Verification items for the finished model (mm, model axes). A direction names the side the tool comes from. Coordinates: 2 decimals unless noted, no trailing zeros. Write each loop counter-clockwise with the first axis right and the second up, starting at its lowest first coordinate (ties: lowest second). Pieces come first, ordered by that corner, then holes. Notation, with made-up numbers: (61.25, -18.75) -> (79.25, -18.75) arc R12 cw to (79.25, -11.75) -> close; hole circle Ø11 at (-37, -13.5). An arc over 180 degrees is marked (long way). Answer in a Markdown table with one row per item.
```python
from build123d import *

# Parameters (mm, degrees)
F1_DEPTH = 50.8
F2_R     = 12.7
F4_D     = 12.7


with BuildPart() as f1:
    # F0 (on Top) → F1 (new body)
    with BuildSketch(Plane.XY):
        Polygon((0, 50.8), (0, 0), (152.4, 0), (152.4, 76.2), (101.6, 76.2), (101.6, 50.8), align=None)
    extrude(amount=F1_DEPTH)

    # F2
    f2_edges = [f1.edges().sort_by_distance(p)[0] for p in [
        (0, 25.4, 0),
        (76.2, 0, 0),
        (152.4, 38.1, 0),
        (127, 76.2, 0),
        (101.6, 63.5, 0),
        (50.8, 50.8, 0),
        (152.4, 0, 25.4),
        (0, 0, 25.4),
        (0, 50.8, 25.4),
        (152.4, 76.2, 25.4),
    ]]
    fillet(f2_edges, radius=F2_R)

    # F4 (through all)
    with Locations(Plane.XY.offset(50.8)):
        with Locations((50.8, 25.4), (101.6, 25.4)):
            Hole(F4_D / 2)


solid = f1.part
```
1. Sectioned sample at A-A, the plane y = 25.4. Record the cut outline in (x, z), and give its area (3 significant figures).
Findings below:
| item | result |
|---|---|
| outline | (0, 12.7) arc R12.7 ccw to (12.7, 0) -> (44.45, 0) -> (44.45, 50.8) -> (0, 50.8) -> close; (57.15, 0) -> (95.25, 0) -> (95.25, 50.8) -> (57.15, 50.8) -> close; (107.95, 0) -> (139.7, 0) arc R12.7 ccw to (152.4, 12.7) -> (152.4, 50.8) -> (107.95, 50.8) -> close |
| area | 6,380 mm² |
2. Go/stop test with flat-tipped pins: pin 1 (2 mm diameter, centred on x = 135, z = 7.5, fed in from +Y); pin 2 (20.5 mm diameter, centred on x = 101.6, y = 25.4, fed in from +Z); pin 3 (12 mm diameter, centred on y = 58.5, z = 41.5, fed in from -X). Record where each tip stops, or that it passes through.
Findings below:
| item | result |
|---|---|
| pin 1 | stops at y = 75.49 |
| pin 2 | stops at z = 50.8 |
| pin 3 | stops at x = 101.6 |
3. Sectioned sample at D-D, the plane x = 27.5. Record the cut outline in (y, z), and give its area (3 significant figures).
Findings below:
| item | result |
|---|---|
| outline | (0, 12.7) arc R12.7 ccw to (12.7, 0) -> (38.1, 0) arc R12.7 ccw to (50.8, 12.7) -> (50.8, 50.8) -> (0, 50.8) -> close |
| area | 2,510 mm² |
4. Access from +Z, -Z, +X, -X, +Y, -Y to the whole of each face (thin tool, end or side, straight path). Record for faces 1 (the face through (0, 26, 31)), 2 (the face through (62.79, 47.18, 3.82)), 3 (the face through (101.6, 64, 31)).
Findings below:
| item | result |
|---|---|
| face 1 | +Z, -Z, -X, +Y, -Y |
| face 2 | -Z, -X, +Y |
| face 3 | +Z, -Z, -X, +Y |
5. Release check for a two-part mould opening along X. For faces 4 (the face through (107.944, 25.679, 25.044)), 5 (the face through (148.78, 72.38, 32.02)), 6 (the face through (44.934, 22.968, 25.044)), 7 (the face through (3.62, 3.82, 32.02)) record: released by +X, released by -X, zero draft, split by the parting line, or undercut.
Findings below:
| item | result |
|---|---|
| face 4 | undercut |
| face 5 | released by +X |
| face 6 | undercut |
| face 7 | released by -X |
6. Sectioned sample at B-B, the plane x = 50.8. Record the cut outline in (y, z), and give its area (3 significant figures).
Findings below:
| item | result |
|---|---|
| outline | (0, 12.7) arc R12.7 ccw to (12.7, 0) -> (19.05, 0) -> (19.05, 50.8) -> (0, 50.8) -> close; (31.75, 0) -> (38.1, 0) arc R12.7 ccw to (50.8, 12.7) -> (50.8, 50.8) -> (31.75, 50.8) -> close |
| area | 1,870 mm² |
7. Material ranges on probe 1 along X at (y, z) = (25, 22); probe 2 along X at (y, z) = (23, 18); probe 3 along Y at (x, z) = (50.8, 13), recorded low to high. Write a range as from..to.
Findings below:
| item | result |
|---|---|
| probe 1 | x = 0..44.46, 57.14..95.26, 107.94..152.4 |
| probe 2 | x = 0..44.92, 56.68..95.72, 107.48..152.4 |
| probe 3 | y = 0..19.05, 31.75..50.8 |
8. Sectioned sample at C-C, the plane z = 14.5. Record the cut outline in (x, y).
Findings below:
| item | result |
|---|---|
| outline | (0, 12.7) arc R12.7 ccw to (12.7, 0) -> (139.7, 0) arc R12.7 ccw to (152.4, 12.7) -> (152.4, 63.5) arc R12.7 ccw to (139.7, 76.2) -> (101.6, 76.2) -> (101.6, 50.8) -> (12.7, 50.8) arc R12.7 ccw to (0, 38.1) -> close; hole circle Ø12.7 at (50.8, 25.4); hole circle Ø12.7 at (101.6, 25.4) |
